from build123d import *

# Parameters (mm, degrees)
SKETCH1_W                   = 76.2
SKETCH1_H                   = 63.5
BOSS_EXTRUDE1_DEPTH         = 19.05
SKETCH2_W                   = 55.88
SKETCH2_H                   = 63.5
CUT_EXTRUDE1_DEPTH          = 13.97
F_1_4_20_TAPPED_HOLE1_D     = 5.1054
F_1_4_20_TAPPED_HOLE1_DEPTH = 19.05
F_1_4_20_TAPPED_HOLE1_TIP   = 1.533816902
LPATTERN1_COUNT             = 2
LPATTERN1_PITCH             = 57.15
LPATTERN1_COUNT_DIR2        = 2
LPATTERN1_PITCH_DIR2        = 66.04


with BuildPart() as part:
    # Sketch1 → Boss-Extrude1 (new body)
    with BuildSketch(Plane(origin=(0, 0, 0), x_dir=(0, 0, -1), z_dir=(1, 0, 0))):
        Rectangle(SKETCH1_W, SKETCH1_H)
    extrude(amount=BOSS_EXTRUDE1_DEPTH)

    # Sketch2 → Cut-Extrude1 (cut)
    with BuildSketch(Plane(origin=(19.05, 0, 0), x_dir=(0, 0, -1), z_dir=(1, 0, 0))):
        Rectangle(SKETCH2_W, SKETCH2_H)
    extrude(amount=-CUT_EXTRUDE1_DEPTH, mode=Mode.SUBTRACT)

    # Sketch5 → #10-32 Tapped Hole1 (revolve, cut)
    with BuildSketch(Plane(origin=(19.05, 28.575, 33.02), x_dir=(0, 0, -1), z_dir=(0, 1, 0))):
        Polygon((0, 0), (0, 14.929317848), (2.0193, 13.716), (2.0193, 0), align=None)
    f_10_32_tapped_hole1 = revolve(axis=Axis((25.4, 28.575, 33.02), (-1, 0, 0)), mode=Mode.SUBTRACT)

    # 1/4-20 Tapped Hole1
    with Locations(Plane(origin=(5.08, 0, 0), x_dir=(0, 0, -1), z_dir=(1, 0, 0))):
        with Locations((0, 9.525)):
            Hole(F_1_4_20_TAPPED_HOLE1_D / 2, depth=F_1_4_20_TAPPED_HOLE1_DEPTH)
            with Locations((0, 0, -(F_1_4_20_TAPPED_HOLE1_DEPTH + F_1_4_20_TAPPED_HOLE1_TIP / 2))):  # 118° drill point
                Cone(0, F_1_4_20_TAPPED_HOLE1_D / 2, F_1_4_20_TAPPED_HOLE1_TIP, mode=Mode.SUBTRACT)

    # LPattern1: 10-32 Tapped Hole1 2 × 2
    with Locations(*[(0, -i * LPATTERN1_PITCH, -j * LPATTERN1_PITCH_DIR2) for i in range(LPATTERN1_COUNT) for j in range(LPATTERN1_COUNT_DIR2) if (i, j) != (0, 0)]):
        add(f_10_32_tapped_hole1, mode=Mode.SUBTRACT)


solid = part.part
Geometry: final body of the model. Coordinates: model frame, mm. A direction names the side the tool comes from. Give positions to 0.01 mm unless a question says otherwise; leave off trailing zeros. Loops run counter-clockwise (first coordinate to the right, second up) from the corner with the lowest first, then second, coordinate; pieces in that order, holes last. Notation, with made-up numbers: M 30.5,5.25 L 55.5,5.25 A5 cw 55.5,13.25 Z; hole C 52.5,38.5 d1. An arc over 180 degrees is marked long. Put each result on its own line as item: value. Start each with the question number.
1) Ray query, line 1 along Y through (x, z) = (12, 33.02); line 2 along Z through (x, y) = (13.25, 10.5); line 3 along Z through (x, y) = (10, 27). Return the intervals inside material, ascending.
2) Contact query for flat-ended pins moving along their axis: pin 1 (4 mm diameter, centred on x = 6.5, z = -18.5, fed in from +Y); pin 2 (12 mm diameter, centred on y = 0.5, z = -9, fed in from +X); pin 3 (3 mm diameter, centred on y = 9.525, z = 0, fed in from +X). Output: stop coordinate, or through.
3) Pull-direction query (Y, two-part tool) for faces 4 (the flat face through (3, 31.75, 1)), 5 (the cylindrical face through (12.288, -27.802, 31.155)), 6 (the flat face through (5.08, 0, 0)); classes: pulls with the +Y half, pulls with the -Y half, needs draft (parallel to the pull), parting line crosses it, or undercut.
4) Cut plane B-B (z = 0). Output: boundary loops of the cut face in (x, y), then the cut area to 3 significant figures.
5) Cut plane C-C (y = 5). Output: boundary loops of the cut face in (x, z), then the cut area to 3 significant figures.
6) Cut plane A-A (x = 15.5). Output: boundary loops of the cut face in (y, z) (3 decimals).
7) Access query for faces 1 (the flat face through (12, 0, 27.94)), 2 (the flat face through (19.05, 0, 33)), 3 (the cylindrical face through (12.288, 27.968, 31.094)). Directions: +Z, -Z, +X, -X, +Y, -Y. A direction counts if a zero-diameter tool reaches every point of the face in a straight line with its end or side. Return the directions, or none.
Verdict:
1. line 1: -31.75 to -30.59, -26.56 to 26.56, 30.59 to 31.75
1. line 2: -38.1 to -27.94, 27.94 to 38.1
1. line 3: -38.1 to -34.28, -31.76 to -27.94, 27.94 to 31.76, 34.28 to 38.1
2. pin 1: y = 31.75
2. pin 2: x = 5.08
2. pin 3: through
3. face 4: pulls with the +Y half
3. face 5: undercut
3. face 6: needs draft
4. outline: M 0,-31.75 L 5.08,-31.75 L 5.08,6.97 L 0,6.97 Z; M 0,12.08 L 5.08,12.08 L 5.08,31.75 L 0,31.75 Z
4. area: 297 mm2
5. outline: M 0,-38.1 L 19.05,-38.1 L 19.05,-27.94 L 5.08,-27.94 L 5.08,27.94 L 19.05,27.94 L 19.05,38.1 L 0,38.1 Z
5. area: 671 mm2
6. outline: M -31.75,-38.1 L 31.75,-38.1 L 31.75,-27.94 L -31.75,-27.94 Z; M -31.75,27.94 L 31.75,27.94 L 31.75,38.1 L -31.75,38.1 Z; hole C -28.575,-33.02 d4.039; hole C -28.575,33.02 d4.039; hole C 28.575,-33.02 d4.039; hole C 28.575,33.02 d4.039
7. face 1: +X, +Y, -Y
7. face 2: +Z, -Z, +X, +Y, -Y
7. face 3: +X
